from build123d import *

# Parameters (mm, degrees)
SM_BASE_FLANGE_1_DEPTH = 700
SKETCH_2_R             = 3.5
CUT_EXTRUDE_1_DEPTH    = 5


# Sheet-metal steps are written as plain solids
with BuildPart() as part:
    # Sketch 1 → Базовая кромка1 (new body)
    with BuildSketch(Plane.XY):
        with BuildLine():
            Line((69.782473476, 200), (43.415186116, 200))
            ThreePointArc((43.415186116, 200), (40.476259854, 199.045084972), (38.659903534, 196.545084972))
            Line((38.659903534, 196.545084972), (14.561776314, 122.37867555))
            ThreePointArc((14.561776314, 122.37867555), (14.455209294, 122.000817397), (14.378617193, 121.615762903))
            Line((14.378617193, 121.615762903), (1.672637328, 41.393363285))
            ThreePointArc((1.672637328, 41.393363285), (1.626492362, 41.003486439), (1.611079031, 40.61119096))
            Line((1.611079031, 40.61119096), (1.611079031, -40.61119096))
            ThreePointArc((1.611079031, -40.61119096), (1.626492362, -41.003486439), (1.672637328, -41.393363285))
            Line((1.672637328, -41.393363285), (14.378617193, -121.615762903))
            ThreePointArc((14.378617193, -121.615762903), (14.455209294, -122.000817397), (14.561776314, -122.37867555))
            Line((14.561776314, -122.37867555), (37.544374419, -193.111839379))
            ThreePointArc((37.544374419, -193.111839379), (36.639549016, -196.320108259), (33.329233371, -196.711909935))
            Line((33.329233371, -196.711909935), (8.597245129, -184.110332509))
            Line((8.597245129, -184.110332509), (7.68926413, -185.892345557))
            Line((7.68926413, -185.892345557), (32.421252372, -198.493922983))
            ThreePointArc((32.421252372, -198.493922983), (37.938445112, -197.84092019), (39.446487452, -192.493805391))
            Line((39.446487452, -192.493805391), (16.463889347, -121.760641561))
            ThreePointArc((16.463889347, -121.760641561), (16.399949135, -121.53392667), (16.353993874, -121.302893973))
            Line((16.353993874, -121.302893973), (3.648014009, -41.080494355))
            ThreePointArc((3.648014009, -41.080494355), (3.62032703, -40.846568247), (3.611079031, -40.61119096))
            Line((3.611079031, -40.61119096), (3.611079031, 40.61119096))
            ThreePointArc((3.611079031, 40.61119096), (3.62032703, 40.846568247), (3.648014009, 41.080494355))
            Line((3.648014009, 41.080494355), (16.353993874, 121.302893973))
            ThreePointArc((16.353993874, 121.302893973), (16.399949135, 121.53392667), (16.463889347, 121.760641561))
            Line((16.463889347, 121.760641561), (40.562016567, 195.927050983))
            ThreePointArc((40.562016567, 195.927050983), (41.651830359, 197.427050983), (43.415186116, 198))
            Line((43.415186116, 198), (69.782473476, 198))
            Line((69.782473476, 198), (69.782473476, 200))
        make_face()
    extrude(amount=SM_BASE_FLANGE_1_DEPTH)

    # Зеркальное отражение1: part across plane


with BuildPart() as part_1:
    add(part.part)
    add(part.part.mirror(Plane(origin=(34.691204871, -194.038890362, 0), x_dir=(1, 0, 0), z_dir=(0, 0, 1))))

    # Sketch 2 → Вырез-Вытянуть1 (cut)
    with BuildSketch(Plane(origin=(-20.892826899, -6.788490969, 0), x_dir=(0, 0, -1), z_dir=(0.9510565162951543, 0.3090169943749452, 0))):
        with Locations(Location((-690, -180.2560263, 0), (0, 0, 90))):
            Circle(SKETCH_2_R)
        with Locations(Location((-552, -180.2560263, 0), (0, 0, 90))):
            Circle(SKETCH_2_R)
        with Locations(Location((-414, -180.2560263, 0), (0, 0, 90))):
            Circle(SKETCH_2_R)
        with Locations(Location((-276, -180.2560263, 0), (0, 0, 90))):
            Circle(SKETCH_2_R)
        with Locations(Location((-138, -180.2560263, 0), (0, 0, 90))):
            Circle(SKETCH_2_R)
        with Locations(Location((0, -180.2560263, 0), (0, 0, 90))):
            Circle(SKETCH_2_R)
        with Locations(Location((690, -180.2560263, 0), (0, 0, 90))):
            Circle(SKETCH_2_R)
        with Locations(Location((552, -180.2560263, 0), (0, 0, 90))):
            Circle(SKETCH_2_R)
        with Locations(Location((414, -180.2560263, 0), (0, 0, 90))):
            Circle(SKETCH_2_R)
        with Locations(Location((276, -180.2560263, 0), (0, 0, 90))):
            Circle(SKETCH_2_R)
        with Locations(Location((138, -180.2560263, 0), (0, 0, 90))):
            Circle(SKETCH_2_R)
    extrude(amount=-CUT_EXTRUDE_1_DEPTH, mode=Mode.SUBTRACT)


solid = part_1.part
Work out the finished part from the listing and answer in its coordinate system (mm). A direction names the side the tool comes from. Coordinates: 2 decimals unless noted, no trailing zeros. Loops run counter-clockwise (first coordinate to the right, second up) from the corner with the lowest first, then second, coordinate; pieces in that order, holes last. Notation, with made-up numbers: (-21, 27) -> (6, 27) arc R12 cw to (6, 32) -> close; hole circle Ø8 at (11.5, 64). An arc over 180 degrees is marked (long way). Write each question's results on one line, items separated by ' | '. Start each with the question number.
1) Flat-ended cylindrical pins translate along their axes: P1, Ø1.5, axis at y = -1, z = -269.5, coming from the +X side; P2, Ø21, axis at x = 61, z = -236.5, coming from the -Y side; P3, Ø10, axis at y = -119.5, z = 388, coming from the +X side. Find the tip coordinate at first contact, or state that the pin passes through.
2) Find section B-B on x = 54. Determine the outline of the cut face in (y, z).
3) Find section C-C on y = 143. Determine the outline of the cut face in (x, z), then the cut area to 3 significant figures.
4) Find section A-A on z = -95. Determine the outline of the cut face in (x, y), then the cut area to 3 significant figures.
5) The mould has two halves that part along X. Classify faces 4 (the flat face through (21.14, -190.5, 9.8)), 5 (the flat face through (56, 198, 10)), 6 (the flat face through (10.09, -81.75, 9.8)): pulls with the +X half, pulls with the -X half, needs draft (parallel to the pull), parting line crosses it, or undercut.
6) For faces 1 (the flat face through (7.937, -80.943, 9.8)), 2 (the flat face through (3.611, -1, 10)), 3 (the flat face through (57, 200, 10)), determine the directions among +Z, -Z, +X, -X, +Y, -Y from which every point of the face is accessible in a straight line to the end or side of a thin tool.
7) Consider line 1 along Y through (x, z) = (55.5, 610.5); line 2 along X through (y, z) = (-121, -419.5); line 3 along X through (y, z) = (-36, -3). Determine where each line is inside the solid, lowest interval first.
Response values:
1) P1: stops at x = 3.61 | P2: stops at y = 198 | P3: stops at x = 17.35
2) outline: (198, -700) -> (200, -700) -> (200, 700) -> (198, 700) -> close
3) outline: (21.26, -700) -> (23.36, -700) -> (23.36, 700) -> (21.26, 700) -> close | area: 2,940 mm^2
4) outline: (1.61, -40.61) arc R5 ccw to (1.67, -41.39) -> (14.38, -121.62) arc R5 ccw to (14.56, -122.38) -> (37.54, -193.11) arc R3 cw to (33.33, -196.71) -> (8.6, -184.11) -> (7.69, -185.89) -> (32.42, -198.49) arc R5 ccw to (39.45, -192.49) -> (16.46, -121.76) arc R3 cw to (16.35, -121.3) -> (3.65, -41.08) arc R3 cw to (3.61, -40.61) -> (3.61, 40.61) arc R3 cw to (3.65, 41.08) -> (16.35, 121.3) arc R3 cw to (16.46, 121.76) -> (40.56, 195.93) arc R3 cw to (43.42, 198) -> (69.78, 198) -> (69.78, 200) -> (43.42, 200) arc R5 ccw to (38.66, 196.55) -> (14.56, 122.38) arc R5 ccw to (14.38, 121.62) -> (1.67, 41.39) arc R5 ccw to (1.61, 40.61) -> close | area: 934 mm^2
5) face 4: undercut | face 5: needs draft | face 6: pulls with the +X half
6) face 1: +Z, -Z, -X | face 2: +Z, -Z, +X | face 3: +Z, -Z, +X, -X, +Y
7) line 1: y = 198 to 200 | line 2: x = 14.28 to 16.31 | line 3: x = 1.61 to 3.61
